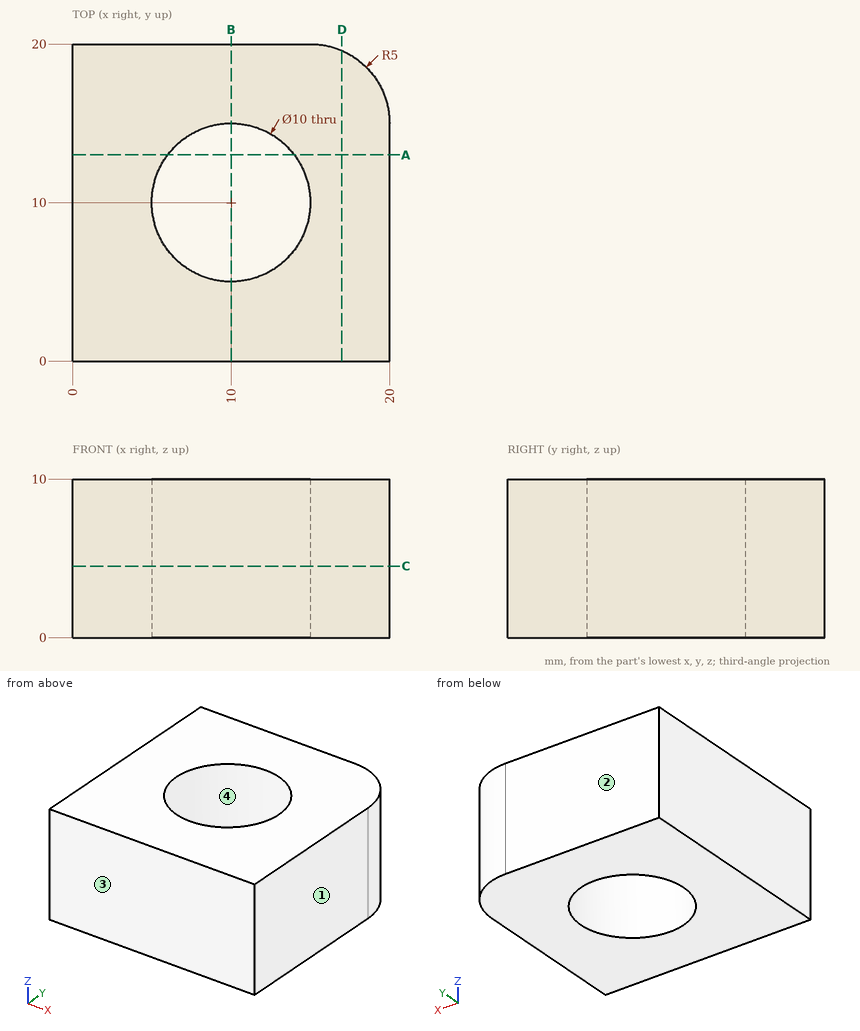
Drawing for the job (mm, zero at the part's lowest x, y, z). Round coordinates to 2 decimals unless told otherwise and drop trailing zeros. Loops run counter-clockwise (first coordinate to the right, second up) from the corner with the lowest first, then second, coordinate; pieces in that order, holes last. Notation, with made-up numbers: (-18.75, 74.25) - (21.25, 74.25) arc R29 cw to (21.25, 97.25) - close; hole circle Ø7 at (-8, 29). An arc over 180 degrees is marked (long way). Return JSON: item names as keys, results as strings. Group by question number.
Q1. Two-plate mould, pull along Y, no slides. Class the marked faces 1, 2, 3 and 4: +Y half, -Y half, draft (parallel to the pull), parting line (faces both ways), or undercut.
Q2. Drill centre lines: line 1 along Y through (x, z) = (10, 2.25); line 2 along Y through (x, z) = (8.5, 9.25); line 3 along X through (y, z) = (14, 3.5). Where is each one in solid material? Low to high. Write a range as [from, to].
Q3. Band-saw the part on B-B on x = 10. Give the cut face in (y, z), plus the area to 3 significant figures.
Q4. Band-saw the part on D-D on x = 17. Give the cut face in (y, z).
Q5. Band-saw the part on C-C on z = 4.5. Give the cut face in (x, y), plus the area to 3 significant figures.
Q6. Band-saw the part on A-A on y = 13. Give the cut face in (x, z).
Solutions:
{
 "1": {"face 1": "draft", "face 2": "+Y half", "face 3": "-Y half", "face 4": "undercut"},
 "2": {"line 1": "y = [0, 5], [15, 20]", "line 2": "y = [0, 5.23], [14.77, 20]", "line 3": "x = [0, 7], [13, 20]"},
 "3": {"outline": "(0, 0) - (5, 0) - (5, 10) - (0, 10) - close; (15, 0) - (20, 0) - (20, 10) - (15, 10) - close", "area": "100 mm^2"},
 "4": {"outline": "(0, 0) - (19.58, 0) - (19.58, 10) - (0, 10) - close"},
 "5": {"outline": "(0, 0) - (20, 0) - (20, 15) arc R5 ccw to (15, 20) - (0, 20) - close; hole circle Ø10 at (10, 10)", "area": "316 mm^2"},
 "6": {"outline": "(0, 0) - (6, 0) - (6, 10) - (0, 10) - close; (14, 0) - (20, 0) - (20, 10) - (14, 10) - close"}
}
